Here's how the part is built. I have some questions about the finished solid (model axes, mm). A direction names the side the tool comes from. Coordinates: 2 decimals unless noted, no trailing zeros. Write each loop counter-clockwise with the first axis right and the second up, starting at its lowest first coordinate (ties: lowest second). Pieces come first, ordered by that corner, then holes. Notation, with made-up numbers: (5, 47.25) -> (61, 47.25) arc R15 ccw to (61, 68.25) -> close; hole circle Ø7 at (58.25, -17). An arc over 180 degrees is marked (long way). Put each result on its own line as item: value. Start each with the question number.
Item 1: For pin 1 (1 mm diameter, centred on x = 0.5, z = 0, fed in from -Y); pin 2 (0.5 mm diameter, centred on x = 0, y = 7, fed in from +Z); pin 3 (0.5 mm diameter, centred on y = 7.5, z = -0.5, fed in from +X); pin 4 (0.9 mm diameter, centred on y = 6.5, z = 0.5, fed in from -X), each with a flat end and sliding along its axis, tell me the tip position at first contact or that it passes through.
Item 2: I want a section at B-B, the plane x = 0. List the corners of the cut face in (y, z) for me, then the cut area to 3 significant figures.
Item 3: On a 3-axis mill with a long thin cutter (end or side, diameter ignored), from which of +Z, -Z, +X, -X, +Y, -Y can I reach the whole of each face in a straight line? I mean faces 1 (the face through (0, 7, -0.9)), 2 (the face through (0, 7, 0.9)), 3 (the face through (0.9, 7, 0)), 4 (the face through (-0.9, 7, 0)). Say none if no direction works.
Item 4: I want a section at D-D, the plane y = 7. List the corners of the cut face in (x, z) for me.
Item 5: I want a section at A-A, the plane z = 0. List the corners of the cut face in (x, y) for me.
Item 6: I need wall thicknesses on line 1 (Z direction, x = -0.7, y = 7.75); line 2 (Y direction, x = 0, z = 1.1). Which ranges of each line are inside material? Lowest first, please. Write a range as [from, to].
Item 7: I want a section at C-C, the plane y = 3.25. List the corners of the cut face in (x, z) for me.
from build123d import *

# Parameters (mm, degrees)
SKETCH1_R           = 1.4
BOSS_EXTRUDE1_DEPTH = 6
SKETCH2_W           = 0.9
SKETCH2_H           = 0.9
BOSS_EXTRUDE2_DEPTH = 2


with BuildPart() as part:
    # Sketch1 → Boss-Extrude1 (new body)
    with BuildSketch(Plane(origin=(0, 0, 0), x_dir=(1, 0, 0), z_dir=(0, 1, 0))):
        with Locations(Location((0, 0, 0), (0, 0, 270))):
            Circle(SKETCH1_R)
    extrude(amount=BOSS_EXTRUDE1_DEPTH)

    # Sketch2 → Boss-Extrude2 (add)
    with BuildSketch(Plane(origin=(0, 6, 0), x_dir=(1, 0, 0), z_dir=(0, 1, 0))):
        with Locations((-0.45, 0.45)):
            Rectangle(SKETCH2_W, SKETCH2_H)
        with Locations((-0.45, -0.45)):
            Rectangle(SKETCH2_W, SKETCH2_H)
        with Locations((0.45, 0.45)):
            Rectangle(SKETCH2_W, SKETCH2_H)
        with Locations((0.45, -0.45)):
            Rectangle(SKETCH2_W, SKETCH2_H)
    extrude(amount=BOSS_EXTRUDE2_DEPTH)


solid = part.part
Calculated:
1. pin 1: stops at y = 0
1. pin 2: stops at z = 0.9
1. pin 3: stops at x = 0.9
1. pin 4: stops at x = -0.9
2. outline: (0, -1.4) -> (6, -1.4) -> (6, -0.9) -> (8, -0.9) -> (8, 0.9) -> (6, 0.9) -> (6, 1.4) -> (0, 1.4) -> close
2. area: 20.4 mm2
3. face 1: -Z, +X, -X, +Y
3. face 2: +Z, +X, -X, +Y
3. face 3: +Z, -Z, +X, +Y
3. face 4: +Z, -Z, -X, +Y
4. outline: (-0.9, -0.9) -> (0.9, -0.9) -> (0.9, 0.9) -> (-0.9, 0.9) -> close
5. outline: (-1.4, 0) -> (1.4, 0) -> (1.4, 6) -> (0.9, 6) -> (0.9, 8) -> (-0.9, 8) -> (-0.9, 6) -> (-1.4, 6) -> close
6. line 1: z = [-0.9, 0.9]
6. line 2: y = [0, 6]
7. outline: circle Ø2.8 at (0, 0)
